Model file for the job. Use its own axes, mm. A direction names the side the tool comes from. Coordinates: 2 decimals unless noted, no trailing zeros. Write each loop counter-clockwise with the first axis right and the second up, starting at its lowest first coordinate (ties: lowest second). Pieces come first, ordered by that corner, then holes. Notation, with made-up numbers: M 85.25,74 L 117.25,74 A25 ccw 117.25,103 Z; hole C 45.25,44.5 d3. An arc over 180 degrees is marked long. Put each result on its own line as item: value. Start each with the question number.
Q1. Pull direction Z, two halves, no side cores. Call faces 4 (the flat face through (-33.99, 1.48, -0.85)), 5 (the flat face through (-35.026, 1.479, -4.305)), 6 (the flat face through (-44.719, 1.479, 9.756)): pulls with the +Z half, pulls with the -Z half, needs draft (parallel to the pull), parting line crosses it, or undercut.
Q2. Which spindle directions (+Z, -Z, +X, -X, +Y, -Y) get a long thin tool onto all of the face, cutting with end or side? Do faces 1 (the flat face through (-40.12, 1.479, 1.863)), 2 (the flat face through (-41.627, 1.479, 8.4)), 3 (the flat face through (-33.23, 1.48, -4.1)). Say none if no direction does.
Q3. Cut at A-A (x = 2). Write the cut outline in (y, z), then the cut area to 3 significant figures.
Q4. Drop flat-ended pins along their axis: pin 1 (1.5 mm diameter, centred on x = -21.5, z = 2.5, fed in from -Y); pin 2 (1 mm diameter, centred on y = 1.5, z = 7.5, fed in from -X); pin 3 (1.5 mm diameter, centred on x = -12, y = 1.5, fed in from -Z). Give the stop position or say it passes through.
Q5. Cut at C-C (x = -18). Write the cut outline in (y, z).
Q6. Drill centre lines: line 1 along X through (y, z) = (0.75, -0.75); line 2 along Z through (x, y) = (-20.5, 1.75); line 3 along X through (y, z) = (2.35, -3.5). Where is each one in solid material? Low to high.
Q7. Cut at B-B (y = 0.85). Write the cut outline in (x, z), then the cut area to 3 significant figures.
```python
from build123d import *

# Parameters (mm, degrees)
SKETCH1_R           = 2.5
SKETCH1_R_2         = 0.5
BOSS_EXTRUDE1_DEPTH = 3


with BuildPart() as part:
    # Sketch1 → Boss-Extrude1 (new body)
    with BuildSketch(Plane(origin=(0, 0, 0), x_dir=(1, 0, 0), z_dir=(0, 1, 0))):
        with BuildLine():
            Line((-33.358616029, 1.612959212), (-34.632118724, 0.070820799))
            Line((-34.632118724, 0.070820799), (-36.945326344, 1.981074841))
            Line((-36.945326344, 1.981074841), (-38.218829039, 0.438936428))
            Line((-38.218829039, 0.438936428), (-35.905621419, -1.471317615))
            Line((-35.905621419, -1.471317615), (-37.179124114, -3.013456028))
            Line((-37.179124114, -3.013456028), (-39.492331734, -1.103201985))
            Line((-39.492331734, -1.103201985), (-40.765834429, -2.645340399))
            Line((-40.765834429, -2.645340399), (-38.452626808, -4.555594441))
            Line((-38.452626808, -4.555594441), (-39.726129503, -6.097732855))
            Line((-39.726129503, -6.097732855), (-42.039337123, -4.187478812))
            Line((-42.039337123, -4.187478812), (-43.312839818, -5.729617226))
            Line((-43.312839818, -5.729617226), (-40.999632198, -7.639871268))
            Line((-40.999632198, -7.639871268), (-42.273134893, -9.182009681))
            Line((-42.273134893, -9.182009681), (-44.586342513, -7.271755639))
            Line((-44.586342513, -7.271755639), (-45.859845208, -8.813894052))
            Line((-45.859845208, -8.813894052), (-43.546637588, -10.724148095))
            ThreePointArc((-43.546637588, -10.724148095), (-17.222782933, -18.730729797), (6.992336159, -5.66632465))
            ThreePointArc((6.992336159, -5.66632465), (5.66632465, 6.992336159), (-6.992336159, 5.66632465))
            ThreePointArc((-6.992336159, 5.66632465), (-19.015227456, -0.820198185), (-32.085113334, 3.155097626))
            Line((-32.085113334, 3.155097626), (-34.398320954, 5.065351668))
            Line((-34.398320954, 5.065351668), (-35.671823649, 3.523213255))
            Line((-35.671823649, 3.523213255), (-33.358616029, 1.612959212))
        make_face()
        with Locations(Location((0, 0, 0), (0, 0, 270))):
            Circle(SKETCH1_R, mode=Mode.SUBTRACT)
        with Locations(Location((-5.06424038, -3.382538894, 0), (0, 0, 270))):
            Circle(SKETCH1_R_2, mode=Mode.SUBTRACT)
        with Locations(Location((-8.39050664, -5.604239317, 0), (0, 0, 270))):
            Circle(SKETCH1_R_2, mode=Mode.SUBTRACT)
    extrude(amount=BOSS_EXTRUDE1_DEPTH)


solid = part.part
```
Computed values:
1. face 4: undercut
1. face 5: pulls with the -Z half
1. face 6: pulls with the +Z half
2. face 1: -Z, -X, +Y, -Y
2. face 2: +Y, -Y
2. face 3: -Z, +Y, -Y
3. outline: M 0,-8.77 L 3,-8.77 L 3,-1.5 L 0,-1.5 Z; M 0,1.5 L 3,1.5 L 3,10.71 L 0,10.71 Z
3. area: 49.5 mm2
4. pin 1: y = 0
4. pin 2: x = -45.19
4. pin 3: z = -1.87
5. outline: M 0,0.69 L 3,0.69 L 3,18.8 L 0,18.8 Z
6. line 1: -37.96 to -35.45, -34.07 to -28.27, -13.29 to -2.38, 2.38 to 8.97
6. line 2: 0.91 to 18.91
6. line 3: -35.64 to -32.5, -9.08 to 8.29
7. outline: M -45.86,8.81 L -44.59,7.27 L -42.27,9.18 L -41,7.64 L -43.31,5.73 L -42.04,4.19 L -39.73,6.1 L -38.45,4.56 L -40.77,2.65 L -39.49,1.1 L -37.18,3.01 L -35.91,1.47 L -38.22,-0.44 L -36.95,-1.98 L -34.63,-0.07 L -33.36,-1.61 L -35.67,-3.52 L -34.4,-5.07 L -32.09,-3.16 A17.75 cw -6.99,-5.67 A9 ccw 6.99,5.67 A35.75 ccw -43.55,10.72 Z; hole C -8.39,5.6 d1; hole C -5.06,3.38 d1; hole C 0,0 d5
7. area: 897 mm2
